Can you work these out from the model? Positions are in its coordinate system, mm. A direction names the side the tool comes from. Give positions to 0.01 mm unless a question says otherwise; leave off trailing zeros. Order: outer loops, then holes, each group sorted by start corner. A loop starts at its lowest first (then second) coordinate and runs counter-clockwise, first axis right, second up. Notation, with made-up numbers: M 48,71.25 L 91,71.25 A24 cw 91,83.25 Z; hole C 62.5,-24.5 d6. An arc over 180 degrees is marked long. Use one line per item in the form item = value. Start each with the question number.
1. I want a section at B-B, the plane z = 7. List the corners of the cut face in (x, y) for me, and give its area (3 significant figures).
2. I need wall thicknesses on L1, parallel to Y at x = 0, z = 3.9; L2, parallel to X at y = -25.5, z = 4; L3, parallel to X at y = -26, z = 2.5. Which ranges of each line are inside material? Lowest first, please.
3. Will these pins go through, and if not, where does the flat tip stop? P1, Ø2.5, axis at x = -13, y = 24.5, coming from the +Z side; P2, Ø4, axis at x = -23.5, z = 3.5, coming from the -Y side; P3, Ø1.2, axis at x = 15.5, z = 4, coming from the -Y side.
4. I want a section at D-D, the plane z = 4. List the corners of the cut face in (x, y) for me.
5. For faces 1 (the face through (20, -26, 4)), 2 (the face through (-1.73, -20.31, 5.54)), 3 (the face through (15, 26, 7)), 4 (the face through (-13, -24, 4)), which set-ups out of +Z, -Z, +X, -X, +Y, -Y let a thin tool reach every point of the face, with its end or its side?
6. I want a section at C-C, the plane x = 0. List the corners of the cut face in (y, z) for me, and give its area (3 significant figures).
7. We'd pull the mould along X, two halves only. Please class faces 5 (the face through (18.4, 23.3, 5.3)), 6 (the face through (13.95, 21.5, 6.99)), 7 (the face through (-23, -23.5, 4)): +X half, -X half, draft (parallel to the pull), parting line (faces both ways), or undercut.
8. I want a section at A-A, the plane y = -12.5. List the corners of the cut face in (x, z) for me, and give its area (3 significant figures).
```python
from build123d import *

# Parameters (mm, degrees)
BOSS_EXTRU_1_DEPTH      = 8
ESQUISSE2_R             = 2
ENL_V_MAT_EXTRU_1_DEPTH = 10
ESQUISSE3_R             = 2
ENL_V_MAT_EXTRU_2_DEPTH = 39.745967532
CHANFREIN1_SIZE         = 2.5
ESQUISSE4_R             = 8
ENL_V_MAT_EXTRU_3_DEPTH = 5
ESQUISSE5_R             = 3
ENL_V_MAT_EXTRU_4_DEPTH = 39.23937761
ESQUISSE6_W             = 40
ESQUISSE6_H             = 8
ENL_V_MAT_EXTRU_5_DEPTH = 2
CONG_1_R                = 3.5


with BuildPart() as part:
    # Esquisse1 → Boss.-Extru.1 (new body)
    with BuildSketch(Plane.XY):
        Polygon((-25, -23.5), (-20, -23.5), (-20, -28.5), (20, -28.5), (20, -23.5), (25, -23.5), (25, 28.5), (-25, 28.5), align=None)
    extrude(amount=BOSS_EXTRU_1_DEPTH)

    # Esquisse2 → Enlèv. mat.-Extru.1 (cut)
    with BuildSketch(Plane.XZ.offset(28.5)):
        with Locations(Location((-15, 4, 0), (0, 0, 270))):
            Circle(ESQUISSE2_R)
        with Locations(Location((15, 4, 0), (0, 0, 270))):
            Circle(ESQUISSE2_R)
    extrude(amount=-ENL_V_MAT_EXTRU_1_DEPTH, mode=Mode.SUBTRACT)

    # Esquisse3 → Enlèv. mat.-Extru.2 (cut, through all)
    with BuildSketch(Plane.XY.offset(8)):
        with Locations((-20, 24.5)):
            Circle(ESQUISSE3_R)
        with Locations((20, 24.5)):
            Circle(ESQUISSE3_R)
        with Locations((0, 24.5)):
            Circle(ESQUISSE3_R)
    extrude(amount=-ENL_V_MAT_EXTRU_2_DEPTH, mode=Mode.SUBTRACT)

    # Chanfrein1
    # the kernel refuses this chamfer: 2.5 mm, written as the material it takes off along each edge
    with BuildSketch(Plane(origin=(-20, 24.5, 0), x_dir=(1, 0, 0), z_dir=(0, -1, 0))) as chanfrein1_piece_1:
        Polygon((2 + CHANFREIN1_SIZE, 0), (2, CHANFREIN1_SIZE), (2, 0), align=None)
    revolve(axis=Axis((-20, 24.5, 0), (0, 0, 1)), mode=Mode.SUBTRACT)
    with BuildSketch(Plane(origin=(20, 24.5, 0), x_dir=(1, 0, 0), z_dir=(0, -1, 0))) as chanfrein1_piece_2:
        Polygon((2 + CHANFREIN1_SIZE, 0), (2, CHANFREIN1_SIZE), (2, 0), align=None)
    revolve(axis=Axis((20, 24.5, 0), (0, 0, 1)), mode=Mode.SUBTRACT)
    with BuildSketch(Plane(origin=(0, 24.5, 0), x_dir=(1, 0, 0), z_dir=(0, -1, 0))) as chanfrein1_piece_3:
        Polygon((2 + CHANFREIN1_SIZE, 0), (2, CHANFREIN1_SIZE), (2, 0), align=None)
    revolve(axis=Axis((0, 24.5, 0), (0, 0, 1)), mode=Mode.SUBTRACT)

    # Esquisse4 → Enlèv. mat.-Extru.3 (cut)
    with BuildSketch(Plane.XY.offset(8)):
        with Locations((0, -12.5)):
            Circle(ESQUISSE4_R)
    extrude(amount=-ENL_V_MAT_EXTRU_3_DEPTH, mode=Mode.SUBTRACT)

    # Esquisse5 → Enlèv. mat.-Extru.4 (cut, through all)
    with BuildSketch(Plane.XY.offset(3)):
        with Locations((0, -12.5)):
            Circle(ESQUISSE5_R)
    extrude(amount=-ENL_V_MAT_EXTRU_4_DEPTH, mode=Mode.SUBTRACT)

    # Esquisse6 → Enlèv. mat.-Extru.5 (cut)
    with BuildSketch(Plane.XY.offset(8)):
        with Locations((-5, 24.5)):
            Rectangle(ESQUISSE6_W, ESQUISSE6_H)
    extrude(amount=-ENL_V_MAT_EXTRU_5_DEPTH, mode=Mode.SUBTRACT)

    # Congé1
    cong_1_edges = [part.edges().sort_by_distance(p)[0] for p in [
        (15, 20.5, 7),
    ]]
    fillet(cong_1_edges, radius=CONG_1_R)


solid = part.part
```
Check result:
q1.outline = M -25,-23.5 L -20,-23.5 L -20,-28.5 L 20,-28.5 L 20,-23.5 L 25,-23.5 L 25,28.5 L 15,28.5 L 15,24 A3.5 cw 11.5,20.5 L -25,20.5 Z; hole C 0,-12.5 d16; hole C 20,24.5 d4
q1.area = 2,270 mm2
q2.L1 = -28.5 to -20.5, -4.5 to 22.5, 26.5 to 28.5
q2.L2 = -20 to -17, -13 to 13, 17 to 20
q2.L3 = -20 to -16.32, -13.68 to 13.68, 16.32 to 20
q3.P1 = 6
q3.P2 = -23.5
q3.P3 = -18.5
q4.outline = M -25,-23.5 L -20,-23.5 L -20,-28.5 L -17,-28.5 L -17,-18.5 L -13,-18.5 L -13,-28.5 L 13,-28.5 L 13,-18.5 L 17,-18.5 L 17,-28.5 L 20,-28.5 L 20,-23.5 L 25,-23.5 L 25,28.5 L -25,28.5 Z; hole C -20,24.5 d4; hole C 0,-12.5 d16; hole C 0,24.5 d4; hole C 20,24.5 d4
q5.face_1 = +Z, -Z, +X, -Y
q5.face_2 = +Z
q5.face_3 = +Z, -X, +Y
q5.face_4 = -Y
q6.outline = M -28.5,0 L -15.5,0 L -15.5,3 L -20.5,3 L -20.5,8 L -28.5,8 Z; M -9.5,0 L 20,0 L 22.5,2.5 L 22.5,6 L 20.5,6 L 20.5,8 L -4.5,8 L -4.5,3 L -9.5,3 Z; M 26.5,2.5 L 28.5,0.5 L 28.5,6 L 26.5,6 Z
q6.area = 312 mm2
q7.face_5 = undercut
q7.face_6 = -X half
q7.face_7 = draft
q8.outline = M -25,0 L -3,0 L -3,3 L -8,3 L -8,8 L -25,8 Z; M 3,0 L 25,0 L 25,8 L 8,8 L 8,3 L 3,3 Z
q8.area = 302 mm2
